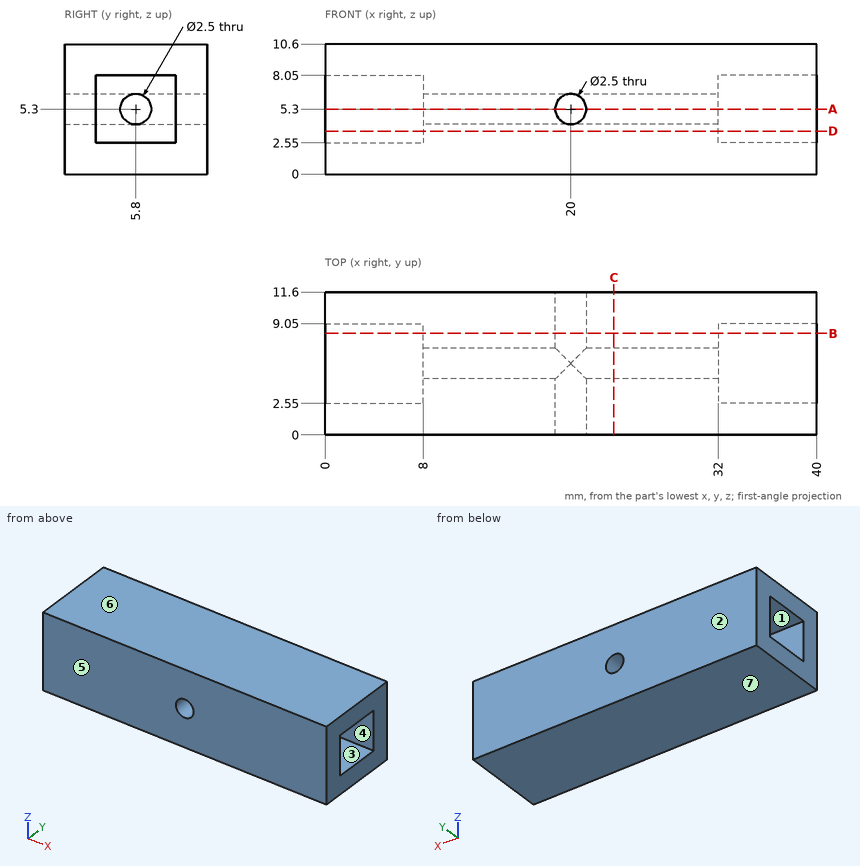
Job drawing, mm, ordinate dimensions from the low corner. One solid piece. A direction names the side the tool comes from. Round coordinates to 2 decimals unless told otherwise and drop trailing zeros. Loops run counter-clockwise (first coordinate to the right, second up) from the corner with the lowest first, then second, coordinate; pieces in that order, holes last. Notation, with made-up numbers: (58.5, 80.25) -> (65.5, 80.25) arc R11 cw to (65.5, 89.25) -> close; hole circle Ø6 at (78.5, 52). An arc over 180 degrees is marked (long way). One line per item, written item: value. Start each with the question number.
Q1. Cut at A-A on z = 5.3. List the corners of the cut face in (x, y).
Q2. Drop flat-ended pins along their axis: pin 1 Ø3 at (y, z) = (5.8, 5.3) entering from +X; pin 2 Ø1.6 at (y, z) = (6.5, 5) entering from -X. Give the stop position or say it passes through.
Q3. Cut at B-B on y = 8.25. List the corners of the cut face in (x, z).
Q4. Cut at C-C on x = 23.5. List the corners of the cut face in (y, z), plus the area to 3 significant figures.
Q5. Two-plate mould, pull along Z, no slides. Class the marked faces 4, 5, 6 and 7: released by +Z, released by -Z, zero draft, split by the parting line, or undercut.
Q6. 3-axis set-ups, long thin cutter, end or side, ignore diameter. For the marked faces 1, 2 and 3: which of +Z, -Z, +X, -X, +Y, -Y reach the whole face in a straight line?
Q7. Cut at D-D on z = 3.5. List the corners of the cut face in (x, y), plus the area to 3 significant figures.
Q8. Probe line 1 along Z through (x, y) = (22.5, 5.8); line 2 along Y through (x, z) = (7.5, 5); line 3 along X through (y, z) = (9.4, 5.3). List the from-to ranges inside material, lowest first.
Computed:
1. outline: (0, 0) -> (18.75, 0) -> (18.75, 4.55) -> (8, 4.55) -> (8, 2.55) -> (0, 2.55) -> close; (0, 9.05) -> (8, 9.05) -> (8, 7.05) -> (18.75, 7.05) -> (18.75, 11.6) -> (0, 11.6) -> close; (21.25, 0) -> (40, 0) -> (40, 2.55) -> (32, 2.55) -> (32, 4.55) -> (21.25, 4.55) -> close; (21.25, 7.05) -> (32, 7.05) -> (32, 9.05) -> (40, 9.05) -> (40, 11.6) -> (21.25, 11.6) -> close
2. pin 1: x = 32
2. pin 2: x = 8
3. outline: (0, 0) -> (40, 0) -> (40, 2.55) -> (32, 2.55) -> (32, 8.05) -> (40, 8.05) -> (40, 10.6) -> (0, 10.6) -> (0, 8.05) -> (8, 8.05) -> (8, 2.55) -> (0, 2.55) -> close; hole circle Ø2.5 at (20, 5.3)
4. outline: (0, 0) -> (11.6, 0) -> (11.6, 10.6) -> (0, 10.6) -> close; hole circle Ø2.5 at (5.8, 5.3)
4. area: 118 mm²
5. face 4: undercut
5. face 5: zero draft
5. face 6: released by +Z
5. face 7: released by -Z
6. face 1: -X
6. face 2: +Z, -Z, +X, -X, +Y
6. face 3: +X
7. outline: (0, 0) -> (40, 0) -> (40, 2.55) -> (32, 2.55) -> (32, 9.05) -> (40, 9.05) -> (40, 11.6) -> (0, 11.6) -> (0, 9.05) -> (8, 9.05) -> (8, 2.55) -> (0, 2.55) -> close
7. area: 360 mm²
8. line 1: 0 to 4.05, 6.55 to 10.6
8. line 2: 0 to 2.55, 9.05 to 11.6
8. line 3: 0 to 18.75, 21.25 to 40
